Design review of the part built by this model. Coordinates are the model's own, in mm. A direction names the side the tool comes from. Coordinates: 2 decimals unless noted, no trailing zeros. Loops run counter-clockwise (first coordinate to the right, second up) from the corner with the lowest first, then second, coordinate; pieces in that order, holes last.
Q1. Wall thickness on probe 1 along Z at (x, y) = (0, 12); probe 2 along Y at (x, z) = (-6.35, 15); probe 3 along Z at (x, y) = (0, 7): over which ranges is each line inside the solid? List them lowest first.
Q2. Draft analysis for pull direction Z (two halves, no side actions). For faces 4 (the face through (11.317, 4.094, 16.908)), 5 (the face through (-6.89, 27.83, -12.83)), 6 (the face through (-0.553, 9.658, 10.944)), state which applies: released by +Z, released by -Z, zero draft, split by the parting line, or undercut.
Q3. Machinability: for faces 1 (the face through (0.71, 9.66, -14.4)), 2 (the face through (-6.89, 27.83, 12.7)), 3 (the face through (-3, 17, -8.065)), which of the approach directions +Z, -Z, +X, -X, +Y, -Y give a long, thin tool a straight path to every point of the face, cutting with its end or side? Answer none if there is none.
Q4. Add section B-B on y = 12. Give the boundary of the cut face in (x, z).
Q5. Add section A-A on z = 0. Give the boundary of the cut face in (x, y), and give its area (3 significant figures).
Q6. For P1, Ø2, axis at x = 0, z = 0, coming from the +Y side; P2, Ø11, axis at x = 1.5, z = 1, coming from the +Y side; P3, Ø2, axis at x = 0, z = 12.7, coming from the +Y side; P4, Ø3, axis at x = 0, z = -12.7, coming from the -Y side, all flat-tipped, find the tip position at first contact; note any pin that passes through.
Q7. Add section C-C on y = 3. Give the number of separate pieces and of enclosed holes in the cut face, and give its area (3 significant figures).
Autodesk Inventor part; units mm, degrees
ref_plane "YZ Plane" through (0, 0, 0) normal (1, 0, 0) x (0, 1, 0)
ref_plane "XZ Plane" through (0, 0, 0) normal (0, 1, 0) x (-1, 0, 0)
ref_plane "XY Plane" through (0, 0, 0) normal (0, 0, 1) x (1, 0, 0)
sketch "Sketch1" plane through (0, 0, 0) normal (0, 0, 1) x (1, 0, 0)
  line L0 (-12.7, 0) -> (12.7, 0)
  line L1 (12.7, 0) -> (12.7, 4.7625)
  line L2 (12.7, 4.7625) -> (-0.831, 28.5406)
  line L3 (-12.7, 25.4) -> (-12.7, 0)
  arc A0 (-0.831, 28.5406) -> (-12.7, 25.4) centre (-6.35, 25.4) ccw
  circle A1 centre (-6.35, 25.4) radius 2.4892
  point P0 (0, 0)
  point P1 (0, 0)
  dimension "d0" = 25.4
  dimension "d1" = 6.35
  dimension "d2" = 4.7625
  dimension "d3" = 25.4
  dimension "d4" = 4.9784
extrude "Extrusion1" add sketch "Sketch1" along normal mid plane 34.925
sketch "Sketch2" plane through (12.7, 0, 17.4625) normal (1, 0, 0) x (0, 0, -1)
  line L0 (34.925, 4.7625) -> (0, 4.7625)
  line L1 (9.398, 31.75) -> (9.398, 7.9375)
  line L2 (12.573, 4.7625) -> (22.352, 4.7625)
  line L3 (25.527, 7.9375) -> (25.527, 31.75)
  arc A0 (9.398, 7.9375) -> (12.573, 4.7625) centre (12.573, 7.9375) ccw
  arc A1 (22.352, 4.7625) -> (25.527, 7.9375) centre (22.352, 7.9375) ccw
  line L4 (0, 0) -> (34.925, 0) construction
  line L5 (34.925, 31.75) -> (0, 31.75)
  point P0 (17.4625, 0)
  point P1 (17.4625, 4.7625)
  point P2 (17.4625, 0)
  point P3 (12.573, 4.7625)
  point P4 (22.352, 4.7625)
  dimension "d7" = 3.175
  dimension "d8" = 16.129
extrude "Extrusion2" cut sketch "Sketch2" against normal through all
chamfer "Chamfer2" [suppressed]
chamfer "Chamfer3" [suppressed]
fillet "Fillet1" radius 3.175 2 edges at (12.7, 2.3813, 17.4625) (12.7, 2.3813, -17.4625)
sketch "Sketch3" plane through (-12.7, 0, -17.4625) normal (0, -1, 0) x (1, 0, 0)
  line L0 (12.7, 30.1625) -> (12.7, 4.7625) construction
  point P0 (12.7, 17.4625)
  point P1 (12.7, 17.4625)
  point P2 (12.7, 17.4625)
  dimension "d12" = 25.4
  dimension "d37" = 38.1
  dimension "d38" = 25.4
  dimension "d32" = 25.4
  dimension "d33" = 25.4
  dimension "d34" = 50.8
hole "Hole1" at (0, 0, -12.7) at (0, 0, 12.7) at (0, 0, 0) direction (0, 1, 0) diameter 3.683 depth 19.05 tip angle 118
pattern_linear "Rectangular Pattern1" [suppressed]
equation "\"d32\" = d33"
properties part number "Cascade Pulley Block2 (WCP-0298)" material "Aluminum 6061"
Entries:
1. probe 1: z = -17.46 to -14.54, -10.86 to -8.06, 8.06 to 10.86, 14.54 to 17.46
1. probe 2: y = 0 to 22.91, 27.89 to 31.75
1. probe 3: z = -17.46 to -14.54, -10.86 to -7.92, 7.92 to 10.86, 14.54 to 17.46
2. face 4: released by +Z
2. face 5: zero draft
2. face 6: undercut
3. face 1: -Y
3. face 2: +Z, -Z
3. face 3: +X, -X, +Y
4. outline: (-12.7, -17.46) - (8.58, -17.46) - (8.58, -8.06) - (-12.7, -8.06) - close; (-12.7, 8.06) - (8.58, 8.06) - (8.58, 17.46) - (-12.7, 17.46) - close; hole circle Ø3.68 at (0, -12.7); hole circle Ø3.68 at (0, 12.7)
5. outline: (-12.7, 0) - (-1.84, 0) - (-1.84, 4.76) - (-12.7, 4.76) - close; (1.84, 0) - (12.7, 0) - (12.7, 4.76) - (1.84, 4.76) - close
5. area: 103 mm2
6. P1: passes through
6. P2: stops at y = 5.2
6. P3: stops at y = 28.82
6. P4: stops at y = 19.26
7. separate pieces: 1
7. enclosed holes: 3
7. area: 851 mm2
